The model under review builds one solid part; all positions refer to its coordinate system, in mm. A direction names the side the tool comes from. Round coordinates to 2 decimals unless told otherwise and drop trailing zeros. Order: outer loops, then holes, each group sorted by start corner. A loop starts at its lowest first (then second) coordinate and runs counter-clockwise, first axis right, second up.
```python
from build123d import *

# Parameters (mm, degrees)
F1_DEPTH = 5.5
F2_R     = 1.125
F3_DEPTH = 4
F4_R     = 2.74999


# Not quite as in the source:
# - a fillet or chamfer is up to 0.001 mm smaller than in the source, because OpenCascade refuses the exact size


with BuildPart() as f1:
    # F0 (on Front) → F1 (new body)
    with BuildSketch(Plane.XZ):
        Polygon((-12.5, 10), (-12.5, 0), (-8.25, 0), (-8.25, 8), (-4, 8), (-4, 7.5), (5.75, 7.5), (5.75, 8), (8.25, 8), (8.25, 0), (12.5, 0), (12.5, 10), align=None)
    extrude(amount=F1_DEPTH)

    # F2 (on face) → F3 (cut)
    with BuildSketch(Plane(origin=(0, 0, 0), x_dir=(1, 0, 0), z_dir=(0, 0, -1))):
        with Locations((-9.75, 2.75)):
            Circle(F2_R)
        with Locations((9.75, 2.75)):
            Circle(F2_R)
    extrude(amount=-F3_DEPTH, mode=Mode.SUBTRACT)

    # F4 (radius 2.75 in the source; OpenCascade refuses exactly that, so slightly less here)
    f4_edges = [f1.edges().sort_by_distance(p)[0] for p in [
        (-12.5, -5.5, 5),
        (-12.5, 0, 5),
        (12.5, -5.5, 5),
        (12.5, 0, 5),
    ]]
    fillet(f4_edges, radius=F4_R)


solid = f1.part
```
(1) Consider section A-A (z = 7.75). State how many separate pieces and enclosed holes the cut face has, and give its area (3 significant figures).
Data:
separate pieces: 3
enclosed holes: 0
area: 93.9 mm2
(2) Insertion check: pin 1 (1.2 mm diameter, centred on x = 6.5, y = -3, fed in from -Z); pin 2 (0.6 mm diameter, centred on y = -3.5, z = 8, fed in from +X); pin 3 (0.7 mm diameter, centred on x = 10, y = -3, fed in from -Z). Each pin has a flat end and moves straight along its axis. Give the tip position at first contact, or say it passes through.
Data:
pin 1: stops at z = 8
pin 2: stops at x = 12.46
pin 3: stops at z = 4
(3) Consider section D-D (x = 6.25). Write out the cut boundary in (y, z).
Data:
outline: (-5.5, 8) - (0, 8) - (0, 10) - (-5.5, 10) - close
(4) For faces 1 (the cylindrical face through (10.823, -3.088, 1.972)), 2 (the flat face through (-11, -2, 0)), 3 (the flat face through (7, -3, 8)), list the 3-axis set-ups (+Z, -Z, +X, -X, +Y, -Y) from which the entire face can be reached by the end or side of a thin tool; tool diameter is ignored.
Data:
face 1: -Z
face 2: -Z, +X, -X, +Y, -Y
face 3: -Z, +Y, -Y
(5) Draft analysis for pull direction Y (two halves, no side actions). For faces 4 (the cylindrical face through (-8.677, -3.088, 1.972)), 5 (the cylindrical face through (-11.72, -4.67, 4.93)), 6 (the flat face through (1, -3, 7.5)), state which applies: pulls with the +Y half, pulls with the -Y half, needs draft (parallel to the pull), parting line crosses it, or undercut.
Data:
face 4: undercut
face 5: pulls with the -Y half
face 6: needs draft
(6) To check wall thickness, follow probe 1 along X at (y, z) = (-2.75, 2.75) (3 decimals); probe 2 along X at (y, z) = (-2.75, 5.75); probe 3 along Y at (x, z) = (-9.75, 2.7) (3 decimals). State the ranges of each line that lie inside material, in increasing order.
Data:
probe 1: x = -12.5 to -10.875, -8.625 to -8.25, 8.25 to 8.625, 10.875 to 12.5
probe 2: x = -12.5 to -8.25, 8.25 to 12.5
probe 3: y = -5.5 to -3.875, -1.625 to 0
